Answer from the drawing. Dimensions are ordinates in mm from the lowest x, y and z of the part. A direction names the side the tool comes from. Give positions to 0.01 mm unless a question says otherwise; leave off trailing zeros. Loops run counter-clockwise (first coordinate to the right, second up) from the corner with the lowest first, then second, coordinate; pieces in that order, holes last. Notation, with made-up numbers: (8.25, 57) -> (37.25, 57) arc R32 ccw to (37.25, 96) -> close; hole circle Ø5 at (51.25, 34.5). An arc over 180 degrees is marked (long way). Write each question's results on one line, items separated by ' | '. Start each with the question number.
Item 1: Each of these flat-tipped pins is pushed along its axis until it touches: P1, Ø4, axis at x = 45.5, y = 28, coming from the +Z side (1 decimal); P2, Ø10, axis at x = 51.5, y = 25, coming from the +Z side (1 decimal); P3, Ø17.5, axis at y = 21, z = 29.5, coming from the +X side (1 decimal). Where does it stop, or does it pass through?
Item 2: Section B-B on z = 29 is taken. Write down the section's boundary in (x, y), and give its area (3 significant figures).
Item 3: Section C-C on y = 15 is taken. Write down the section's boundary in (x, z) (1 decimal), and give its area (3 significant figures).
Item 4: Section D-D on x = 40 is taken. Write down the section's boundary in (y, z), and give its area (3 significant figures).
Item 5: Find the intervals of material crossed by line 1 (Z direction, x = 17, y = 9.5); line 2 (Z direction, x = 49, y = 15); line 3 (Z direction, x = 45.5, y = 4), in increasing order.
Item 6: Section A-A on x = 47.5 is taken. Write down the section's boundary in (y, z).
Item 7: Which of the six approach directions +Z, -Z, +X, -X, +Y, -Y give full straight-line access (tool end or side, diameter ignored) to the marked faces 1 and 2?
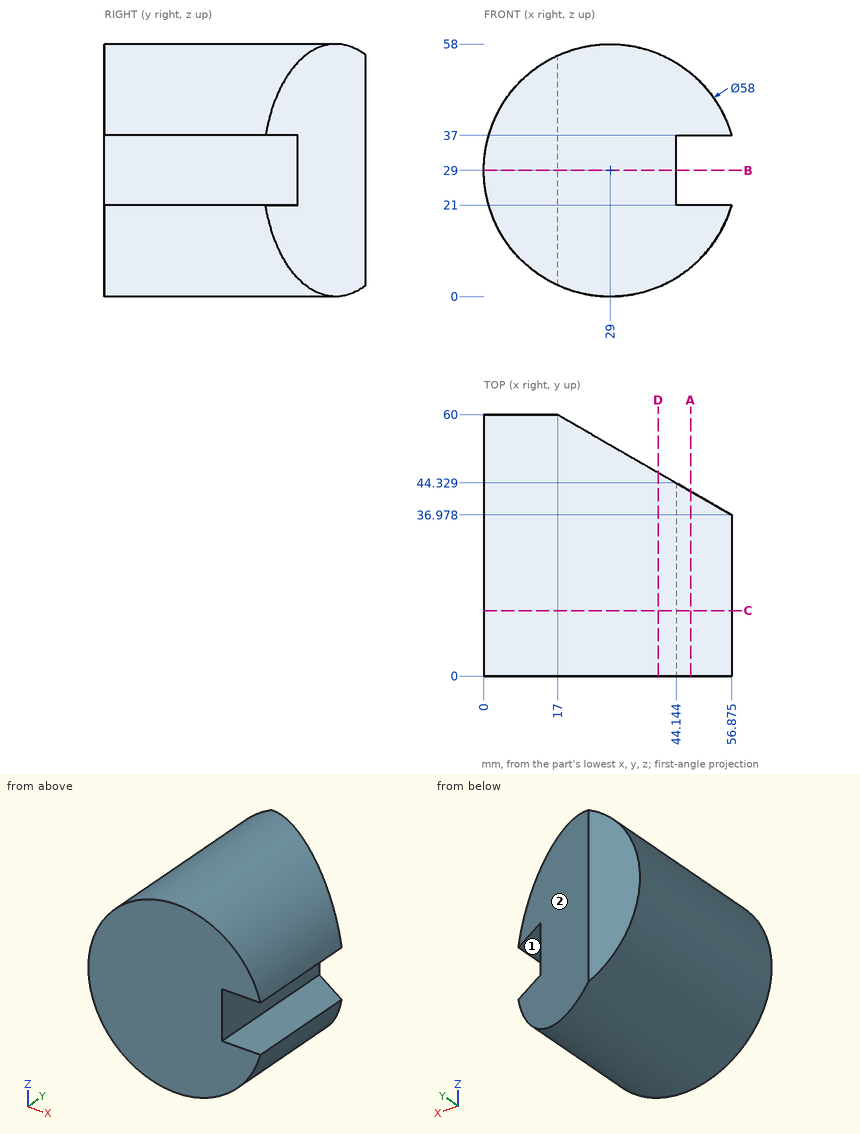
Findings:
1) P1: z = 54.1 | P2: z = 52.1 | P3: x = 56.9
2) outline: (0, 0) -> (44.14, 0) -> (44.14, 44.33) -> (17, 60) -> (0, 60) -> close | area: 2,440 mm2
3) outline: (44.1, 21) -> (44.1, 37) -> (56.9, 37) arc R29 ccw (long way) to (56.9, 21) -> close | area: 2,430 mm2
4) outline: (0, 2.17) -> (46.72, 2.17) -> (46.72, 55.83) -> (0, 55.83) -> close | area: 2,510 mm2
5) line 1: 2.6 to 55.4 | line 2: 8 to 21, 37 to 50 | line 3: 5.15 to 21, 37 to 52.85
6) outline: (0, 6.67) -> (42.39, 6.67) -> (42.39, 21) -> (0, 21) -> close; (0, 37) -> (42.39, 37) -> (42.39, 51.33) -> (0, 51.33) -> close
7) face 1: +X, +Y, -Y | face 2: +Z, -Z, +X, +Y
